```python
from build123d import *

# Parameters (mm, degrees)
F0_R      = 52.201743604
F1_DEPTH  = 300
F3_R      = 25.4
F4_DEPTH  = 152.4
F6_R      = 44.45
F7_DEPTH  = 152.4
F8_R      = 52.201743604
F8_R_2    = 25.4
F9_DEPTH  = 228.6
F13_R     = 31.75
F13_R_2   = 19.05
F15_R     = 31.75
F15_R_2   = 19.05
F14_R     = 31.75
F14_R_2   = 19.05
F16_DEPTH = 10.16
F18_DEPTH = 35.56


with BuildPart() as f1:
    # F0 (on Front) → F1 (new body)
    with BuildSketch(Plane.XZ):
        Circle(F0_R)
    extrude(amount=-F1_DEPTH)

    # F3 (on offset) → F4 (cut)
    with BuildSketch(Plane.XY.offset(63.5)):
        Circle(F3_R)
    extrude(amount=-F4_DEPTH, mode=Mode.SUBTRACT)

    # F6 (on offset) → F7 (cut)
    with BuildSketch(Plane.YZ.offset(63.5)):
        with Locations((-12.7, -50.8)):
            Circle(F6_R)
        with Locations((-12.7, 50.8)):
            Circle(F6_R)
    extrude(amount=-F7_DEPTH, mode=Mode.SUBTRACT)

    # F8 (on face) → F9 (cut)
    with BuildSketch(Plane(origin=(0, 300, 0), x_dir=(-1, 0, 0), z_dir=(0, 1, 0))):
        Circle(F8_R)
        Circle(F8_R_2, mode=Mode.SUBTRACT)
    extrude(amount=-F9_DEPTH, mode=Mode.SUBTRACT)

    # F13 (on offset) + F15 (on offset) + F14 (on offset) → F16 (cut)
    with BuildSketch(Plane(origin=(0, 122.2, 0), x_dir=(-1, 0, 0), z_dir=(0, 1, 0))):
        Circle(F13_R)
        Circle(F13_R_2, mode=Mode.SUBTRACT)
    with BuildSketch(Plane(origin=(0, 173, 0), x_dir=(-1, 0, 0), z_dir=(0, 1, 0))):
        Circle(F15_R)
        Circle(F15_R_2, mode=Mode.SUBTRACT)
    with BuildSketch(Plane(origin=(0, 223.8, 0), x_dir=(-1, 0, 0), z_dir=(0, 1, 0))):
        Circle(F14_R)
        Circle(F14_R_2, mode=Mode.SUBTRACT)
    extrude(amount=-F16_DEPTH, mode=Mode.SUBTRACT)

    # F17 (on face) → F18 (cut)
    with BuildSketch(Plane(origin=(0, 300, 0), x_dir=(-1, 0, 0), z_dir=(0, 1, 0))):
        with BuildLine():
            Line((-24.8980583787, -5.0246083398), (-16.8004676557, 19.050046891))
            ThreePointArc((-16.8004676557, 19.050046891), (-24.0746552308, 8.097590723), (-24.8980583787, -5.0246083398))
        make_face()
        with BuildLine():
            Line((-16.8004676557, 19.050046891), (8.097590723, 24.0746552308))
            ThreePointArc((8.097590723, 24.0746552308), (-5.0246083398, 24.8980583787), (-16.8004676557, 19.050046891))
        make_face()
        with BuildLine():
            Line((8.097590723, 24.0746552308), (24.8980583787, 5.0246083398))
            ThreePointArc((24.8980583787, 5.0246083398), (19.050046891, 16.8004676557), (8.097590723, 24.0746552308))
        make_face()
        with BuildLine():
            ThreePointArc((16.8004676557, -19.050046891), (23.1505062413, -10.4505531324), (25.4, 0))
            ThreePointArc((25.4, 0), (25.2742030816, 2.5248086244), (24.8980583787, 5.0246083398))
            Line((24.8980583787, 5.0246083398), (16.8004676557, -19.050046891))
        make_face()
        with BuildLine():
            ThreePointArc((-8.097590723, -24.0746552308), (5.0246083398, -24.8980583787), (16.8004676557, -19.050046891))
            Line((16.8004676557, -19.050046891), (-8.097590723, -24.0746552308))
        make_face()
        with BuildLine():
            ThreePointArc((-24.8980583787, -5.0246083398), (-19.050046891, -16.8004676557), (-8.097590723, -24.0746552308))
            Line((-8.097590723, -24.0746552308), (-24.8980583787, -5.0246083398))
        make_face()
    extrude(amount=-F18_DEPTH, mode=Mode.SUBTRACT)


solid = f1.part
```
Check sheet for the modelled part. Datum: model origin and axes. Units: mm. A direction names the side the tool comes from. Coordinates: 2 decimals unless noted, no trailing zeros. Loops run counter-clockwise (first coordinate to the right, second up) from the corner with the lowest first, then second, coordinate; pieces in that order, holes last. Notation, with made-up numbers: M 52,62 L 65,62 A27 ccw 65,92 Z; hole C 2,-4.75 d6. An arc over 180 degrees is marked long. Answer as a JSON object with one key per item and string values.
1. Sectioned sample at D-D on x = 31.5. Record the cut outline in (y, z).
Outcome:
{"outline": "M 0,-8.2 A44.45 cw 30.79,-41.63 L 71.4,-41.63 L 71.4,41.63 L 30.79,41.63 A44.45 cw 0,8.2 Z"}
2. Sectioned sample at A-A on y = 63. Record the cut outline in (x, z).
Outcome:
{"outline": "C 0,0 d104.4"}
3. Sectioned sample at C-C on z = -41. Record the cut outline in (x, y), and give its area (3 significant figures).
Outcome:
{"outline": "M -32.31,30.66 L 32.31,30.66 L 32.31,71.4 L -32.31,71.4 Z", "area": "2,630 mm²"}
4. Release check for a two-part mould opening along Y. For faces 1 (the flat face through (0, 300, 0)), 2 (the flat face through (-4, 213.64, 19)), 3 (the cylindrical face through (0.722, 26.936, -30.681)) record: pulls with the +Y half, pulls with the -Y half, needs draft (parallel to the pull), parting line crosses it, or undercut.
Outcome:
{"face 1": "pulls with the +Y half", "face 2": "undercut", "face 3": "pulls with the -Y half"}
5. Depth check by flat-ended pin: P1, Ø15, axis at x = 11.5, z = -9, coming from the -Y side; P2, Ø2, axis at y = 214, z = 8.5, coming from the +X side; P3, Ø2, axis at x = 16, z = -37.5, coming from the -Y side. Enter the tip coordinate at first touch or a pass-through.
Outcome:
{"P1": "y = 16.86", "P2": "x = 24.25", "P3": "y = 29.39"}
6. Sectioned sample at B-B on x = -41. Record the cut outline in (y, z).
Outcome:
{"outline": "M 0,-8.2 A44.45 cw 27.72,-32.31 L 71.4,-32.31 L 71.4,32.31 L 27.72,32.31 A44.45 cw 0,8.2 Z"}
7. Access from +Z, -Z, +X, -X, +Y, -Y to the whole of each face (thin tool, end or side, straight path). Record for faces 4 (the flat face through (-16.38, 282.469, 14.683)), 5 (the cylindrical face through (15.12, 218.79, -11.59)), 6 (the cylindrical face through (5.506, 142.804, -24.796)), 7 (the flat face through (4.526, 282.469, 21.527)).
Outcome:
{"face 4": "+Z, -X, +Y", "face 5": "none", "face 6": "+Y", "face 7": "+Z, +X, +Y"}
8. Scan lines: L1, parallel to Y at x = 15.5, z = 12.5; L2, parallel to Y at x = 9.5, z = 20; L3, parallel to Y at x = 30, z = 8. Record each from-to range of solid material in increasing order. Write a range as from..to.
Outcome:
{"L1": "20.12..112.04, 122.2..162.84, 173..213.64, 223.8..300", "L2": "23.56..112.04, 122.2..162.84, 173..213.64, 223.8..300", "L3": "0..71.4"}
